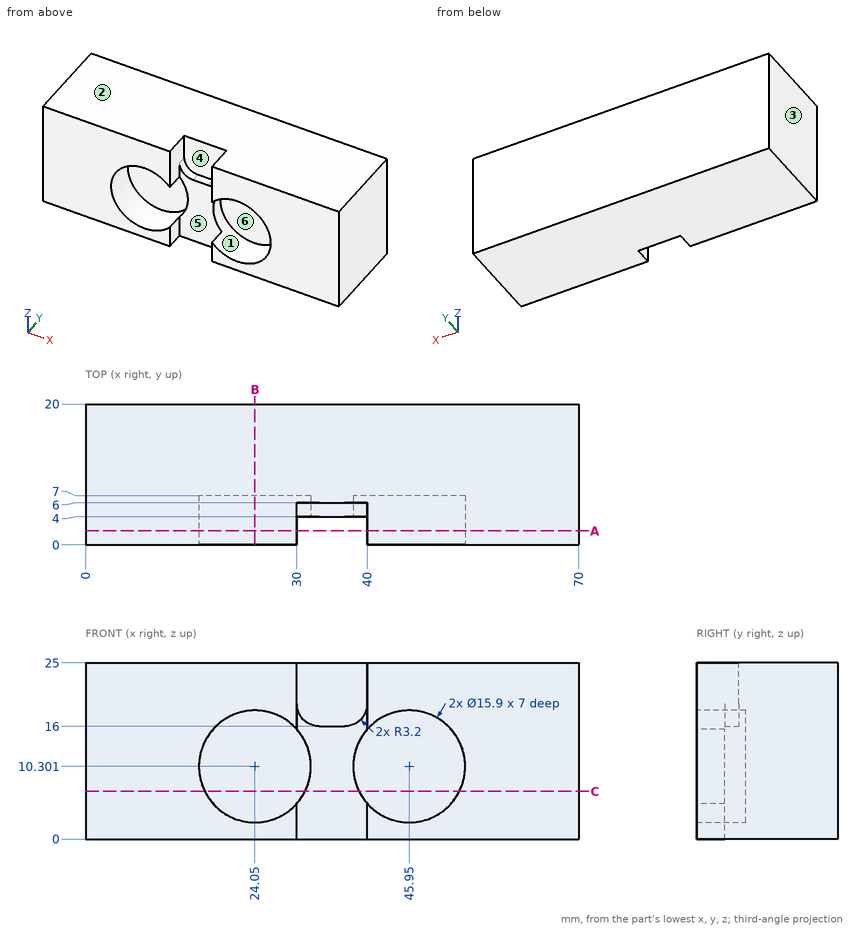
For this review, use the dimensioned drawing (mm, ordinates from the lowest corner) and the shaded views. A direction names the side the tool comes from. Coordinates: 2 decimals unless noted, no trailing zeros. Loops run counter-clockwise (first coordinate to the right, second up) from the corner with the lowest first, then second, coordinate; pieces in that order, holes last. Notation, with made-up numbers: (69.5, 46.5) -> (117.5, 46.5) arc R25 ccw to (117.5, 68.5) -> close; hole circle Ø10 at (-29.5, 32). An arc over 180 degrees is marked (long way). Return JSON: item names as keys, results as strings. Group by question number.
(1) Tool access review of the marked faces 4, 5 and 6: name each direction out of +Z, -Z, +X, -X, +Y, -Y from which nothing blocks a thin tool from reaching the whole face with its end or side.
(2) Consider section C-C, the plane z = 6.75. Give the boundary of the cut face in (x, y).
(3) Consider section B-B, the plane x = 24.05. Give the boundary of the cut face in (y, z).
(4) Mouldability with a two-part tool opening along Z and no side actions: class the marked faces 1, 2 and 3 as pulls with the +Z half, pulls with the -Z half, needs draft (parallel to the pull), parting line crosses it, or undercut.
(5) For pin 1 Ø3 at (x, z) = (37, 7) entering from -Y; pin 2 Ø14.5 at (x, z) = (45.95, 10.3) entering from -Y, all flat-tipped, find the tip position at first contact; note any pin that passes through.
(6) To check wall thickness, follow L1, parallel to X at y = 4.25, z = 11.75; L2, parallel to X at y = 1.5, z = 21.75; L3, parallel to Z at x = 24.05, y = 2.5. State the ranges of each line that lie inside material, in increasing order.
(7) Consider section A-A, the plane y = 2. Give the boundary of the cut face in (x, z), plus the area to 3 significant figures.
Results below:
{
 "1": {"face 4": "+Z, -Y", "face 5": "+Z, -Z, -Y", "face 6": "-Y"},
 "2": {"outline": "(0, 0) -> (16.94, 0) -> (16.94, 7) -> (31.16, 7) -> (31.16, 4) -> (38.84, 4) -> (38.84, 7) -> (53.06, 7) -> (53.06, 0) -> (70, 0) -> (70, 20) -> (0, 20) -> close"},
 "3": {"outline": "(0, 0) -> (20, 0) -> (20, 25) -> (0, 25) -> (0, 18.25) -> (7, 18.25) -> (7, 2.35) -> (0, 2.35) -> close"},
 "4": {"face 1": "undercut", "face 2": "pulls with the +Z half", "face 3": "needs draft"},
 "5": {"pin 1": "stops at y = 4", "pin 2": "stops at y = 7"},
 "6": {"L1": "x = 0 to 16.23, 31.87 to 38.13, 53.77 to 70", "L2": "x = 0 to 30, 40 to 70", "L3": "z = 0 to 2.35, 18.25 to 25"},
 "7": {"outline": "(0, 0) -> (30, 0) -> (30, 5.03) arc R7.95 cw (long way) to (30, 15.57) -> (30, 25) -> (0, 25) -> close; (40, 0) -> (70, 0) -> (70, 25) -> (40, 25) -> (40, 15.57) arc R7.95 cw (long way) to (40, 5.03) -> close", "area": "1,130 mm2"}
}
